CAD build for the part. Positions are in the model's coordinates, mm. A direction names the side the tool comes from. Round coordinates to 2 decimals unless told otherwise and drop trailing zeros. Put each result on its own line as item: value. Start each with the question number.
from build123d import *

# Parameters (mm, degrees)
F0_R     = 19.05
F1_DEPTH = 6.35
F2_D     = 3.81
F3_R     = 12.7
F4_DEPTH = 1.524
F5_R     = 1.52399


# Not quite as in the source:
# - a fillet or chamfer is up to 0.001 mm smaller than in the source, because OpenCascade refuses the exact size


with BuildPart() as f1:
    # F0 (on Top) → F1 (new body)
    with BuildSketch(Plane.XY):
        Circle(F0_R)
    extrude(amount=F1_DEPTH)

    # F2 (through all)
    with Locations(Plane(origin=(0, 0, 0), x_dir=(1, 0, 0), z_dir=(0, 0, -1))):
        with Locations((7.9375, 13.7481532851), (-7.9375, 13.7481532851), (-15.875, 0), (-7.9375, -13.7481532851), (7.9375, -13.7481532851), (15.875, 0)):
            Hole(F2_D / 2)

    # F3 (on face) → F4 (cut)
    with BuildSketch(Plane.XY.offset(6.35)):
        Circle(F3_R)
    extrude(amount=-F4_DEPTH, mode=Mode.SUBTRACT)

    # F5 (radius 1.524 in the source; OpenCascade refuses exactly that, so slightly less here)
    f5_edges = [f1.edges().sort_by_distance(p)[0] for p in [
        (-12.7, 0, 4.826),
    ]]
    fillet(f5_edges, radius=F5_R)


solid = f1.part
(1) Cut at A-A on y = 0. Count the separate pieces of the cut face and the enclosed holes in it, and give its area (3 significant figures).
(2) Tool access for faces 4 (the flat face through (0, 0, 4.826)), 5 (the cylindrical face through (-8.817, 15.438, 3.219)): list every direction of +Z, -Z, +X, -X, +Y, -Y with a clear straight run to the whole face (end or side of a thin tool).
(3) Flat gauge pins, fed straight in: pin 1 Ø2 at (y, z) = (13.5, 4.5) entering from -X; pin 2 Ø1.5 at (x, z) = (2.5, 3) entering from +Y. Where does each tip first touch, or does it go through?
(4) Drill centre lines: line 1 along Y through (x, z) = (8, 1.75); line 2 along Y through (x, z) = (7, 0.75); line 3 along Z through (x, y) = (-3, -10.5). Where is each one in solid material? Low to high.
(5) Mould opens along Y. For faces 1 (the flat face through (4, -12.4, 6.35)), 2 (the cylindrical face through (-15.12, -11.59, 3.13)), 3 (the cylindrical face through (6.12, -14.32, 3.22)) say: +Y half, -Y half, draft (parallel to the pull), parting line (faces both ways), or undercut.
Taken from the geometry:
1. separate pieces: 3
1. enclosed holes: 0
1. area: 156 mm2
2. face 4: +Z
2. face 5: +Z, -Z
3. pin 1: x = -14.38
3. pin 2: y = 18.97
4. line 1: -17.29 to -15.65, -11.84 to 11.84, 15.65 to 17.29
4. line 2: -17.72 to -15.41, -12.09 to 12.09, 15.41 to 17.72
4. line 3: 0 to 4.83
5. face 1: draft
5. face 2: parting line
5. face 3: undercut
